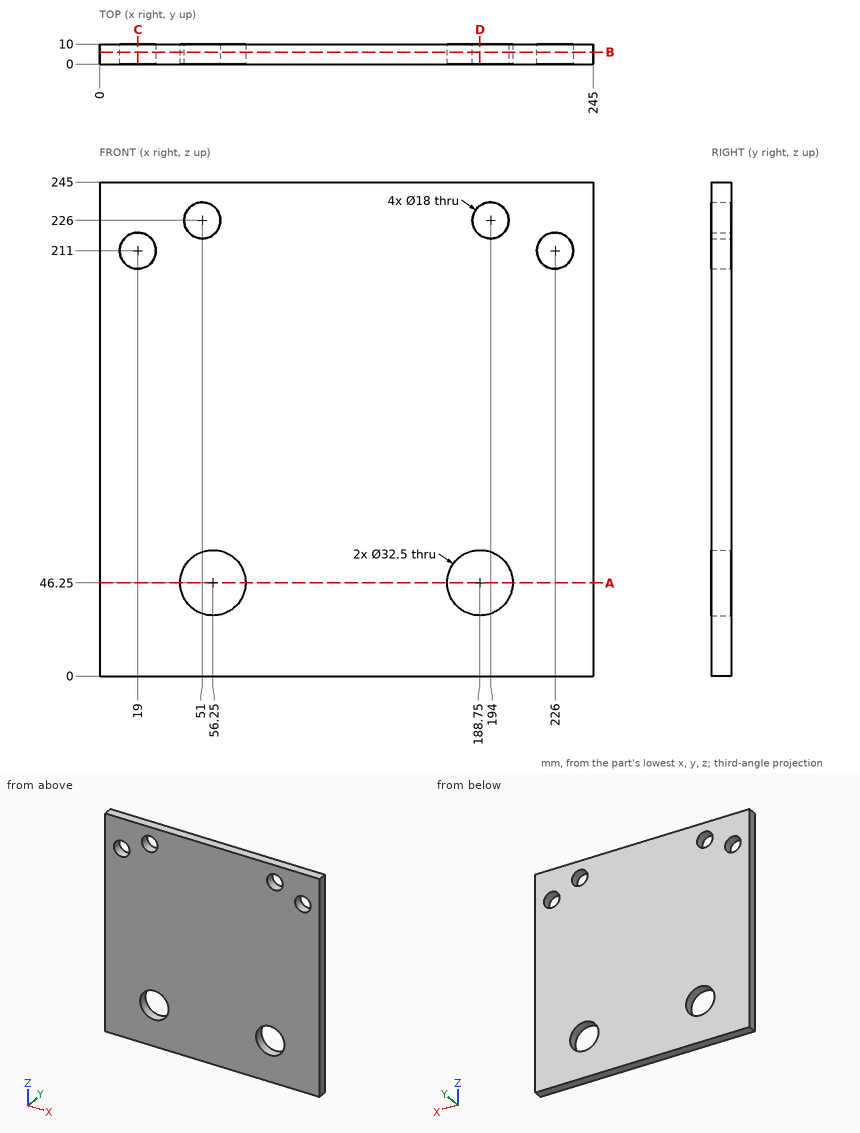
Study the drawing (mm; zero at the part's minimum x, y, z) and answer. Coordinates: 2 decimals unless noted, no trailing zeros. Write each loop counter-clockwise with the first axis right and the second up, starting at its lowest first coordinate (ties: lowest second). Pieces come first, ordered by that corner, then holes. Notation, with made-up numbers: (87, 5) - (101, 5) arc R22 ccw to (101, 12) - close; hole circle Ø4 at (-38.5, -12.75). An arc over 180 degrees is marked (long way). Return JSON: item names as keys, results as strings. Group by question number.
1. A cutting plane is placed at B-B, the plane y = 6. Determine the outline of the cut face in (x, z).
2. Given pin 1 (1 mm diameter, centred on x = 218, y = 8, fed in from -Z); pin 2 (16 mm diameter, centred on x = 51, z = 226, fed in from +Y), each flat-ended and moving along its own axis, determine where each tip first touches the part or whether it passes through.
3. Straight lines are drawn through the part: L1, parallel to X at y = 5.5, z = 226; L2, parallel to X at y = 4, z = 46.25; L3, parallel to Z at x = 19, y = 6.75. For each, find the intervals that lie inside material, in ascending order.
4. A cutting plane is placed at D-D, the plane x = 188.75. Determine the outline of the cut face in (y, z).
5. A cutting plane is placed at C-C, the plane x = 19. Determine the outline of the cut face in (y, z).
6. A cutting plane is placed at A-A, the plane z = 46.25. Determine the outline of the cut face in (x, y).
Ans:
{
 "1": {"outline": "(0, 0) - (245, 0) - (245, 245) - (0, 245) - close; hole circle Ø18 at (19, 211); hole circle Ø32.5 at (56.25, 46.25); hole circle Ø18 at (51, 226); hole circle Ø32.5 at (188.75, 46.25); hole circle Ø18 at (194, 226); hole circle Ø18 at (226, 211)"},
 "2": {"pin 1": "z = 0", "pin 2": "through"},
 "3": {"L1": "0 to 42, 60 to 185, 203 to 245", "L2": "0 to 40, 72.5 to 172.5, 205 to 245", "L3": "0 to 202, 220 to 245"},
 "4": {"outline": "(0, 0) - (10, 0) - (10, 30) - (0, 30) - close; (0, 62.5) - (10, 62.5) - (10, 218.69) - (0, 218.69) - close; (0, 233.31) - (10, 233.31) - (10, 245) - (0, 245) - close"},
 "5": {"outline": "(0, 0) - (10, 0) - (10, 202) - (0, 202) - close; (0, 220) - (10, 220) - (10, 245) - (0, 245) - close"},
 "6": {"outline": "(0, 0) - (40, 0) - (40, 10) - (0, 10) - close; (72.5, 0) - (172.5, 0) - (172.5, 10) - (72.5, 10) - close; (205, 0) - (245, 0) - (245, 10) - (205, 10) - close"}
}
